Verification items for this drawing (mm, ordinates from the low corner). Give positions to 0.01 mm unless a question says otherwise; leave off trailing zeros. Loops run counter-clockwise (first coordinate to the right, second up) from the corner with the lowest first, then second, coordinate; pieces in that order, holes last. Notation, with made-up numbers: (3, -0.5) -> (27, -0.5) arc R19 ccw to (27, 3.5) -> close; hole circle Ø9 at (29.25, 27). An arc over 180 degrees is marked (long way). Answer as a JSON object with one key per item and string values.
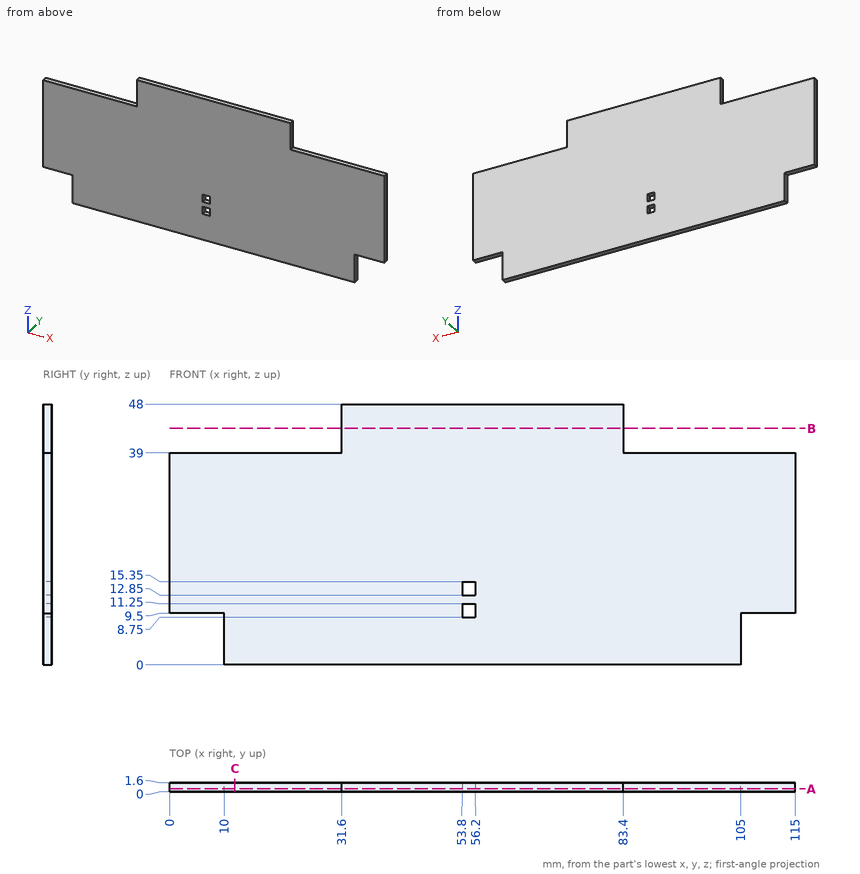
1) Material ranges on line 1 along Z through (x, y) = (104, 0.45); line 2 along X through (y, z) = (1.1, 43); line 3 along X through (y, z) = (1.55, 10), recorded low to high. Write a range as from..to.
Geometry check:
{"line 1": "z = 0..39", "line 2": "x = 31.6..83.4", "line 3": "x = 0..53.8, 56.2..115"}
2) Section check A-A on y = 0.5. Record the cut outline in (x, z), plus the area to 3 significant figures.
Geometry check:
{"outline": "(0, 9.5) -> (10, 9.5) -> (10, 0) -> (105, 0) -> (105, 9.5) -> (115, 9.5) -> (115, 39) -> (83.4, 39) -> (83.4, 48) -> (31.6, 48) -> (31.6, 39) -> (0, 39) -> close; hole (53.8, 8.75) -> (56.2, 8.75) -> (56.2, 11.25) -> (53.8, 11.25) -> close; hole (53.8, 12.85) -> (56.2, 12.85) -> (56.2, 15.35) -> (53.8, 15.35) -> close", "area": "4,750 mm2"}
3) Section check B-B on z = 43.5. Record the cut outline in (x, y), plus the area to 3 significant figures.
Geometry check:
{"outline": "(31.6, 0) -> (83.4, 0) -> (83.4, 1.6) -> (31.6, 1.6) -> close", "area": "82.9 mm2"}
4) Depth check by flat-ended pin: P1, Ø0.8, axis at x = 92.5, y = 1, coming from the +Z side; P2, Ø10, axis at x = 40.5, z = 37.5, coming from the -Y side; P3, Ø0.5, axis at y = 1, z = 44.5, coming from the -X side; P4, Ø0.5, axis at x = 3.5, y = 1, coming from the -Z side. Enter the tip coordinate at first touch or a pass-through.
Geometry check:
{"P1": "stops at z = 39", "P2": "stops at y = 0", "P3": "stops at x = 31.6", "P4": "stops at z = 9.5"}
5) Section check C-C on x = 12. Record the cut outline in (y, z), plus the area to 3 significant figures.
Geometry check:
{"outline": "(0, 0) -> (1.6, 0) -> (1.6, 39) -> (0, 39) -> close", "area": "62.4 mm2"}
